Answer from the drawing. Dimensions are ordinates in mm from the lowest x, y and z of the part. A direction names the side the tool comes from. Coordinates: 2 decimals unless noted, no trailing zeros. Write each loop counter-clockwise with the first axis right and the second up, starting at its lowest first coordinate (ties: lowest second). Pieces come first, ordered by that corner, then holes.
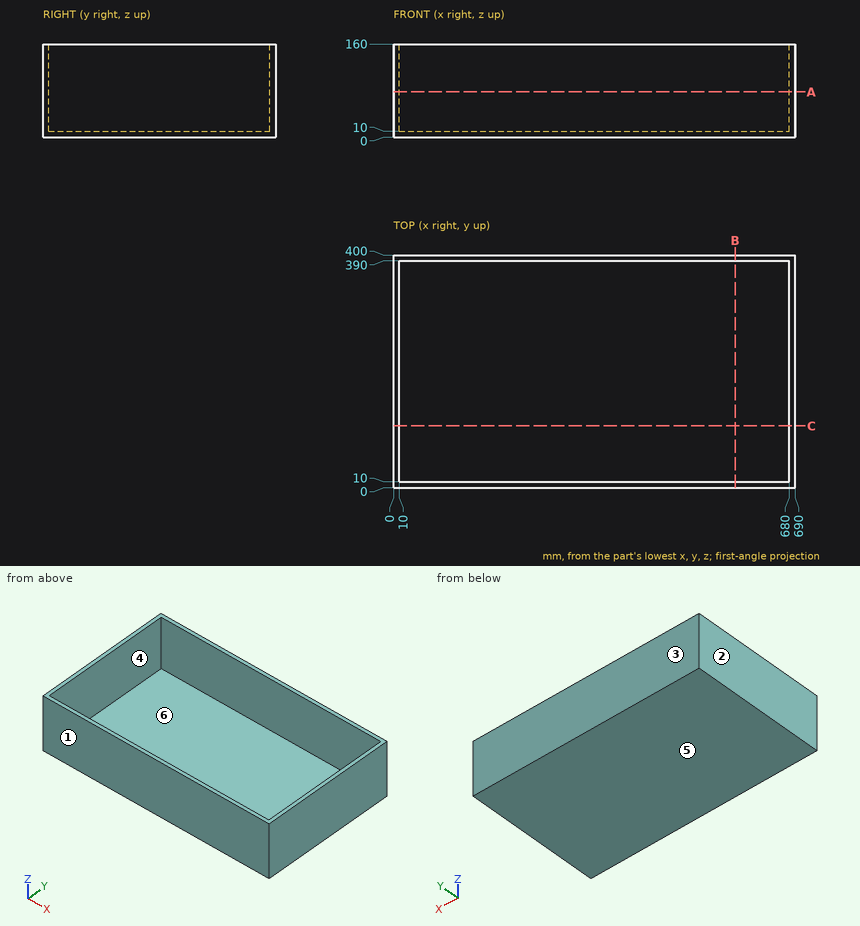
(1) Section A-A, the plane z = 77.5 is taken. Write down the section's boundary in (x, y).
(2) Find the intervals of material crossed by probe 1 along Y at (x, z) = (647, 71.5); probe 2 along X at (y, z) = (286.5, 19); probe 3 along Z at (x, y) = (218.5, 371), in increasing order.
(3) Section B-B, the plane x = 587 is taken. Write down the section's boundary in (y, z), plus the area to 3 significant figures.
(4) Which of the six approach directions +Z, -Z, +X, -X, +Y, -Y give full straight-line access (tool end or side, diameter ignored) to the marked faces 5 and 6?
(5) For a pull along Y with two mould halves and no side action, classify the marked faces 1, 2, 3 and 4 as pulls with the +Y half, pulls with the -Y half, needs draft (parallel to the pull), parting line crosses it, or undercut.
(6) Section C-C, the plane y = 106.5 is taken. Write down the section's boundary in (x, z).
Solution:
1. outline: (0, 0) - (690, 0) - (690, 400) - (0, 400) - close; hole (10, 10) - (680, 10) - (680, 390) - (10, 390) - close
2. probe 1: y = 0 to 10, 390 to 400
2. probe 2: x = 0 to 10, 680 to 690
2. probe 3: z = 0 to 10
3. outline: (0, 0) - (400, 0) - (400, 160) - (390, 160) - (390, 10) - (10, 10) - (10, 160) - (0, 160) - close
3. area: 7,000 mm2
4. face 5: -Z, +X, -X, +Y, -Y
4. face 6: +Z
5. face 1: pulls with the -Y half
5. face 2: needs draft
5. face 3: pulls with the +Y half
5. face 4: undercut
6. outline: (0, 0) - (690, 0) - (690, 160) - (680, 160) - (680, 10) - (10, 10) - (10, 160) - (0, 160) - close
